Geometry: final body of the model. Coordinates: model frame, mm. Round coordinates to 2 decimals unless told otherwise and drop trailing zeros. Order: outer loops, then holes, each group sorted by start corner. A loop starts at its lowest first (then second) coordinate and runs counter-clockwise, first axis right, second up. Notation, with made-up numbers: M 8,14 L 25,14 A31 cw 25,47 Z; hole C -7,11.25 d1. An arc over 180 degrees is marked long. Put each result on its own line as item: value. Start each with the question number.
1) Section A-A, the plane x = 0. Return loops of the section in (y, z), then the cut area to 3 significant figures.
2) Material intervals for probe 1 along X at (y, z) = (3.5, 0); probe 2 along X at (y, z) = (2.95, 33.5); probe 3 along Z at (x, y) = (-3.5, 3.65), sorted ascending. Write a range as [from, to].
3) Section D-D, the plane z = -49.5. Return loops of the section in (x, y), then the cut area to 3 significant figures.
4) First-contact query: P1, Ø5, axis at x = -35, z = 0, coming from the +Y side; P2, Ø2, axis at x = -7, y = 2.5, coming from the -Z side; P3, Ø1.5, axis at y = 1, z = -42.5, coming from the -X side; P4, Ø1.5, axis at x = -23.5, y = 4, coming from the -Z side. Flat tips, straight axial feed; report the tip coordinate or a pass-through.
5) Section C-C, the plane y = 4.1. Count the separate pieces of the cut face and the enclosed holes in it, then the cut area to 3 significant figures.
6) Section B-B, the plane z = 0. Return loops of the section in (x, y), then the cut area to 3 significant figures.
from build123d import *

# Parameters (mm, degrees)
SKETCH_1_R         = 65
SKETCH_1_R_2       = 3
SKETCH_1_R_3       = 10.5
EXTRUDE_3_DEPTH    = 4.917000374
CUT_EXTRUDE1_START = -5.917000374
SKETCH1_R          = 3
CUT_EXTRUDE1_DEPTH = 6.917000374
CIRPATTERN1_COUNT  = 4


with BuildPart() as part:
    # 草圖1 → 填料-伸長3 (new body)
    with BuildSketch(Plane(origin=(0, 0, 0), x_dir=(1, 0, 0), z_dir=(0, 1, 0))):
        Circle(SKETCH_1_R)
        with Locations((-35, 0)):
            Circle(SKETCH_1_R_2, mode=Mode.SUBTRACT)
        with Locations((35, 0)):
            Circle(SKETCH_1_R_2, mode=Mode.SUBTRACT)
        with Locations((0, -35)):
            Circle(SKETCH_1_R_2, mode=Mode.SUBTRACT)
        with Locations((0, 35)):
            Circle(SKETCH_1_R_2, mode=Mode.SUBTRACT)
        Circle(SKETCH_1_R_3, mode=Mode.SUBTRACT)
    extrude(amount=EXTRUDE_3_DEPTH)

    # Sketch1 → Cut-Extrude1 (cut)
    with BuildSketch(Plane(origin=(0, 4.917000374, 0), x_dir=(1, 0, 0), z_dir=(0, 1, 0)).offset(CUT_EXTRUDE1_START)):
        with Locations((-38.890872965, 38.890872965)):
            Circle(SKETCH1_R)
    cut_extrude1 = extrude(amount=CUT_EXTRUDE1_DEPTH, mode=Mode.SUBTRACT)

    # CirPattern1: Cut-Extrude1 ×4 about axis
    cirpattern1_axis = Axis((0, 0, 0), (0, 1, 0))
    for i in range(1, CIRPATTERN1_COUNT):
        add(cut_extrude1.rotate(cirpattern1_axis, i * 360 / CIRPATTERN1_COUNT), mode=Mode.SUBTRACT)


solid = part.part
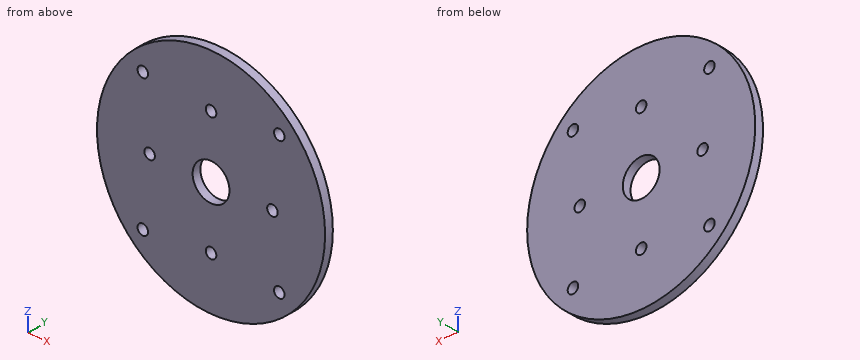
Result sheet:
1. outline: M 0,-65 L 4.92,-65 L 4.92,-38 L 0,-38 Z; M 0,-32 L 4.92,-32 L 4.92,-10.5 L 0,-10.5 Z; M 0,10.5 L 4.92,10.5 L 4.92,32 L 0,32 Z; M 0,38 L 4.92,38 L 4.92,65 L 0,65 Z
1. area: 477 mm2
2. probe 1: x = [-65, -38], [-32, -10.5], [10.5, 32], [38, 65]
2. probe 2: x = [-55.7, -2.6], [2.6, 55.7]
2. probe 3: z = [-64.91, -9.9], [9.9, 64.91]
3. outline: M -42.13,0 L 42.13,0 L 42.13,4.92 L -42.13,4.92 Z
3. area: 414 mm2
4. P1: passes through
4. P2: stops at z = -64.72
4. P3: stops at x = -49.82
4. P4: stops at z = -60.89
5. separate pieces: 1
5. enclosed holes: 9
5. area: 12,700 mm2
6. outline: M -65,0 L -38,0 L -38,4.92 L -65,4.92 Z; M -32,0 L -10.5,0 L -10.5,4.92 L -32,4.92 Z; M 10.5,0 L 32,0 L 32,4.92 L 10.5,4.92 Z; M 38,0 L 65,0 L 65,4.92 L 38,4.92 Z
6. area: 477 mm2
